from build123d import *

# Parameters (mm, degrees)
SKETCH2_W           = 150
SKETCH2_H           = 500
BOSS_EXTRUDE1_DEPTH = 1.5
SKETCH3_R           = 5
BOSS_EXTRUDE2_DEPTH = 1.5


with BuildPart() as part:
    # Sketch2 → Boss-Extrude1 (new body)
    with BuildSketch(Plane.XY):
        Rectangle(SKETCH2_W, SKETCH2_H)
    extrude(amount=BOSS_EXTRUDE1_DEPTH)

    # Sketch3 → Boss-Extrude2 (add)
    with BuildSketch(Plane(origin=(0, 250, 0), x_dir=(1, 0, 0), z_dir=(0, 1, 0))):
        with BuildLine():
            Line((37, 0), (37, 8))
            ThreePointArc((37, 8), (45, 16), (53, 8))
            Line((53, 8), (53, 0))
            Line((53, 0), (37, 0))
        make_face()
        with Locations(Location((45, 8, 0), (0, 0, 270))):
            Circle(SKETCH3_R, mode=Mode.SUBTRACT)
    extrude(amount=-BOSS_EXTRUDE2_DEPTH)


solid = part.part
Read the model definition and answer for the solid it produces. Units are mm, in the model's axes. A direction names the side the tool comes from. Round coordinates to 2 decimals unless told otherwise and drop trailing zeros. Write each loop counter-clockwise with the first axis right and the second up, starting at its lowest first coordinate (ties: lowest second). Pieces come first, ordered by that corner, then holes. Notation, with made-up numbers: (33, 34.5) - (58, 34.5) arc R26 cw to (58, 61.5) - close; hole circle Ø11 at (30.25, 4.25). An arc over 180 degrees is marked (long way). One line per question, with ' | ' between items. Start each with the question number.
1. For faces 4 (the face through (21.9, 250, 0.5)), 5 (the face through (45.1, 248.5, -2.8)), determine the directions among +Z, -Z, +X, -X, +Y, -Y from which every point of the face is accessible in a straight line to the end or side of a thin tool.
2. Section C-C (x = -40.5) is taken. Determine the outline of the cut face in (y, z), and give its area (3 significant figures).
3. Find the intervals of material crossed by probe 1 along X at (y, z) = (248.85, -8); probe 2 along Z at (x, y) = (39, -212.5), in increasing order. Write a range as [from, to].
4. Section B-B (y = 174) is taken. Determine the outline of the cut face in (x, z).
5. Each of these flat-tipped pins is pushed along its axis until it touches: pin 1 (12 mm diameter, centred on x = -29, y = -32.5, fed in from -Z); pin 2 (5 mm diameter, centred on x = 26, z = -4.5, fed in from -Y); pin 3 (1.6 mm diameter, centred on y = 249, z = -3.5, fed in from -X); pin 4 (1.2 mm diameter, centred on y = 249.5, z = -5.5, fed in from +X). Where does it stop, or does it pass through?
6. For a pull along X with two mould halves and no side action, classify faces 1 (the face through (-1, 4, 1.5)), 2 (the face through (45, 249, -16)), 3 (the face through (49, 249, -5)) as +X half, -X half, draft (parallel to the pull), parting line (faces both ways), or undercut.
7. Section A-A (x = 45) is taken. Determine the outline of the cut face in (y, z), and give its area (3 significant figures).
Filled in:
1) face 4: +Z, -Z, +X, -X, +Y | face 5: -Z, +X, -X, -Y
2) outline: (-250, 0) - (250, 0) - (250, 1.5) - (-250, 1.5) - close | area: 750 mm²
3) probe 1: [37, 40], [50, 53] | probe 2: [0, 1.5]
4) outline: (-75, 0) - (75, 0) - (75, 1.5) - (-75, 1.5) - close
5) pin 1: z = 0 | pin 2: through | pin 3: x = 37 | pin 4: x = 53
6) face 1: draft | face 2: parting line | face 3: undercut
7) outline: (-250, 0) - (248.5, 0) - (248.5, -3) - (250, -3) - (250, 1.5) - (-250, 1.5) - close; (248.5, -16) - (250, -16) - (250, -13) - (248.5, -13) - close | area: 759 mm²
